For this review, use the dimensioned drawing (mm, ordinates from the lowest corner) and the shaded views. A direction names the side the tool comes from. Coordinates: 2 decimals unless noted, no trailing zeros. Loops run counter-clockwise (first coordinate to the right, second up) from the corner with the lowest first, then second, coordinate; pieces in that order, holes last. Notation, with made-up numbers: (17.25, 18.25) - (75.25, 18.25) arc R28 ccw to (75.25, 39.25) - close; hole circle Ø2 at (28, 62.5). An arc over 180 degrees is marked (long way). Answer in a Markdown table with one row per item. Add a question column.
(1) We need section A-A, the plane y = 5. Write out the cut boundary in (x, z).
(2) We need section B-B, the plane x = 23.5. Write out the cut boundary in (y, z), plus the area to 3 significant figures.
(3) We need section C-C, the plane z = 20.25. Write out the cut boundary in (x, y), plus the area to 3 significant figures.
(4) For the marked faces 1, 2 and 3, list the 3-axis set-ups (+Z, -Z, +X, -X, +Y, -Y) from which the entire face can be reached by the end or side of a thin tool; tool diameter is ignored.
(5) To check wall thickness, follow L1, parallel to Y at x = 23.5, z = 20.95; L2, parallel to Z at x = 5, y = 32; L3, parallel to Y at x = 13.5, z = 19.75. State the ranges of each line that lie inside material, in increasing order. Write a range as [from, to].
(6) Clearance check with flat-ended pins moving along their axes: pin 1 (2 mm diameter, centred on x = 23.5, y = 5, fed in from -Z); pin 2 (5.5 mm diameter, centred on x = 34.5, y = 5, fed in from -Z); pin 3 (6 mm diameter, centred on y = 34, z = 2.5, fed in from +X); pin 4 (1 mm diameter, centred on y = 32, z = 7, fed in from -X). State where each tip first meets the part, or that it passes through.
(7) We need section D-D, the plane x = 4.75. Write out the cut boundary in (y, z), plus the area to 3 significant figures.
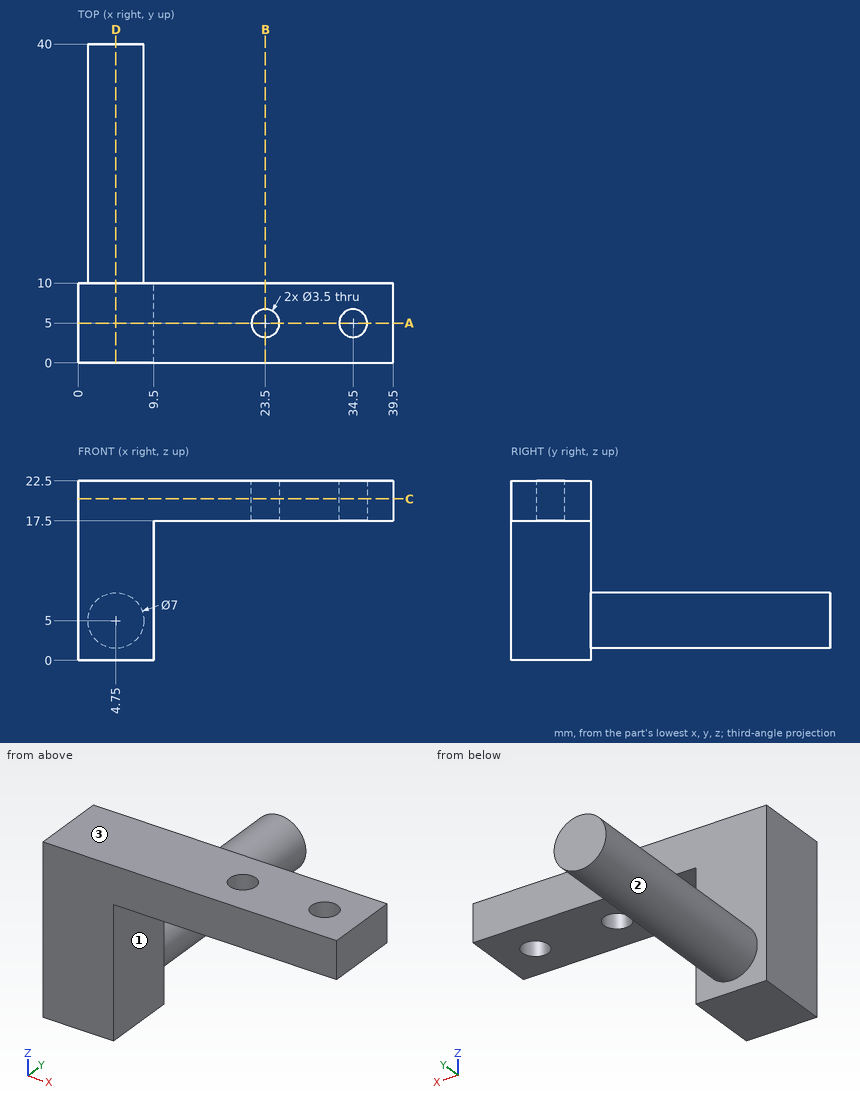
Responses:
| question | item | result |
|---|---|---|
| 1 | outline | (0, 0) - (9.5, 0) - (9.5, 17.5) - (21.75, 17.5) - (21.75, 22.5) - (0, 22.5) - close; (25.25, 17.5) - (32.75, 17.5) - (32.75, 22.5) - (25.25, 22.5) - close; (36.25, 17.5) - (39.5, 17.5) - (39.5, 22.5) - (36.25, 22.5) - close |
| 2 | outline | (0, 17.5) - (3.25, 17.5) - (3.25, 22.5) - (0, 22.5) - close; (6.75, 17.5) - (10, 17.5) - (10, 22.5) - (6.75, 22.5) - close |
| 2 | area | 32.5 mm2 |
| 3 | outline | (0, 0) - (39.5, 0) - (39.5, 10) - (0, 10) - close; hole circle Ø3.5 at (23.5, 5); hole circle Ø3.5 at (34.5, 5) |
| 3 | area | 376 mm2 |
| 4 | face 1 | -Z, +X, +Y, -Y |
| 4 | face 2 | +Y |
| 4 | face 3 | +Z, +X, -X, +Y, -Y |
| 5 | L1 | y = [0, 3.25], [6.75, 10] |
| 5 | L2 | z = [1.51, 8.49] |
| 5 | L3 | y = [0, 10] |
| 6 | pin 1 | passes through |
| 6 | pin 2 | stops at z = 17.5 |
| 6 | pin 3 | stops at x = 8.25 |
| 6 | pin 4 | stops at x = 1.59 |
| 7 | outline | (0, 0) - (10, 0) - (10, 1.5) - (40, 1.5) - (40, 8.5) - (10, 8.5) - (10, 22.5) - (0, 22.5) - close |
| 7 | area | 435 mm2 |
